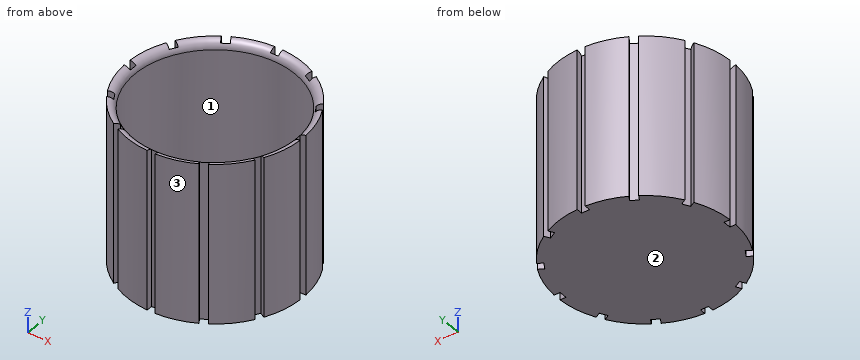
```python
from build123d import *

# Parameters (mm, degrees)
F0_R            = 55
F0_R_2          = 50
F1_DEPTH        = 100
F2_R            = 50
F3_DEPTH        = 1.2
F4_W            = 5
F4_H            = 5
F5_DEPTH        = 200.6
F5_COPIES_COUNT = 12


# Not quite as in the source:
# - a fillet or chamfer that OpenCascade refuses, or shapes differently, is made with other operations: its cross-section is extruded or revolved along the edge and cut away or added
# - a pattern or mirror of a feature is missing from the dataset's text; its kind, count and spacing are read off the source's solid


with BuildPart() as f1:
    # F0 (on Top) → F1 (new body)
    with BuildSketch(Plane.XY):
        Circle(F0_R)
        Circle(F0_R_2, mode=Mode.SUBTRACT)
    extrude(amount=F1_DEPTH)

    # F2 (on Top) → F3 (join)
    with BuildSketch(Plane.XY):
        Circle(F2_R)
    extrude(amount=F3_DEPTH)

    # F4 (on Top) → F5 (cut)
    with BuildSketch(Plane.XY):
        with Locations((0, 53.6743810624)):
            Rectangle(F4_W, F4_H)
    f5 = extrude(amount=F5_DEPTH, mode=Mode.SUBTRACT)

    # F5_copies: F5 ×12 about axis
    f5_copies_axis = Axis((0, 0, 0), (0, 0, 1))
    for i in range(1, F5_COPIES_COUNT):
        add(f5.rotate(f5_copies_axis, i * 360 / F5_COPIES_COUNT), mode=Mode.SUBTRACT)

    # F7: fillet of radius 5 on 1 edges, made by hand

    # F7_s1 → F7_t2 (revolve, cut)
    with BuildSketch(Plane.XZ):
        with BuildLine():
            ThreePointArc((55, 100), (51.4644660941, 98.5355339059), (50, 95))
            Line((50, 95), (50, 100))
            Line((50, 100), (55, 100))
        make_face()
    revolve(axis=Axis((0, 0, 100), (0, 0, 1)), mode=Mode.SUBTRACT)


solid = f1.part
```
Check sheet for the modelled part. Datum: model origin and axes. Units: mm. Face numbers are marked on the shaded views. Round coordinates to 2 decimals unless told otherwise and drop trailing zeros. Order: outer loops, then holes, each group sorted by start corner. A loop starts at its lowest first (then second) coordinate and runs counter-clockwise, first axis right, second up.
1) Go/stop test with flat-tipped pins: pin 1 Ø1.5 at (x, z) = (-15.5, 46.5) entering from -Y; pin 2 Ø2.5 at (x, z) = (-1, 69.5) entering from -Y; pin 3 Ø4 at (x, y) = (-27, 11) entering from +Z. Record where each tip stops, or that it passes through.
2) Section check A-A (y = 0). Record the boundary of the cut face in (x, z).
3) Mould release check, pull along X, two halves, no side actions. Record for the marked faces 1, 2 and 3: +X half, -X half, draft (parallel to the pull), parting line (faces both ways), or undercut.
4) Scan lines: line 1 (Y direction, x = 0, z = 22.5); line 2 (X direction, y = 24.5, z = 38.5); line 3 (Y direction, x = 46, z = 37). Record each from-to range of solid material in increasing order.
Result:
1. pin 1: stops at y = -52.99
1. pin 2: stops at y = -51.17
1. pin 3: stops at z = 1.2
2. outline: (-51.17, 0) - (51.17, 0) - (51.17, 98.22) arc R5 ccw to (50, 95) - (50, 1.2) - (-50, 1.2) - (-50, 95) arc R5 ccw to (-51.17, 98.22) - close
3. face 1: undercut
3. face 2: draft
3. face 3: +X half
4. line 1: y = -51.17 to -50, 50 to 51.17
4. line 2: x = -49.24 to -47.44, -44.95 to -43.59, 43.59 to 44.95, 47.44 to 49.24
4. line 3: y = -30.15 to -29.44, -23.67 to -19.6, 19.6 to 23.67, 29.44 to 30.15
